Part model, mm, in its own coordinate system. A direction names the side the tool comes from. Give positions to 0.01 mm unless a question says otherwise; leave off trailing zeros. Write each loop counter-clockwise with the first axis right and the second up, starting at its lowest first coordinate (ties: lowest second). Pieces come first, ordered by that corner, then holes. Notation, with made-up numbers: (36, 73.25) - (51, 73.25) arc R23 ccw to (51, 84.25) - close; hole circle Ø3 at (72, -11.75). An arc over 180 degrees is marked (long way). Answer in a Markdown table with one row per item. Add a question column.
1. Which spindle directions (+Z, -Z, +X, -X, +Y, -Y) get a long thin tool onto all of the face, cutting with end or side? Do faces 1 (the cylindrical face through (41.727, 76.958, 23.918)), 2 (the cylindrical face through (57.14, 50.1, 19.34)), 3 (the flat face through (42, 47, 12)), 4 (the cylindrical face through (36.86, 50.1, 19.34)). Say none if no direction does.
2. Pull direction X, two halves, no side cores. Call faces 5 (the flat face through (41, 62, 18)), 6 (the cylindrical face through (43, 50, 26)), 7 (the cylindrical face through (36.86, 79.1, 18.18)): released by +X, released by -X, zero draft, split by the parting line, or undercut.
3. Drop flat-ended pins along their axis: pin 1 Ø4 at (y, z) = (55, 14) entering from -X; pin 2 Ø11 at (y, z) = (59, 15.5) entering from +X; pin 3 Ø8 at (x, y) = (48, 58.5) entering from +Z; pin 4 Ø1.8 at (x, y) = (41.5, 75.5) entering from -Z. Give the stop position or say it passes through.
4. Band-saw the part on A-A on z = 22. Write the cut outline in (x, y).
5. Band-saw the part on D-D on y = 56. Write the cut outline in (x, z).
6. Band-saw the part on B-B on x = 42. State how many separate pieces and enclosed holes the cut face has, plus the area to 3 significant figures.
7. Probe line 1 along Y through (x, z) = (54, 10.75); line 2 along X through (y, z) = (76, 10.25); line 3 along Y through (x, z) = (52, 28.5). List the from-to ranges inside material, lowest first.
```python
from build123d import *

# Parameters (mm, degrees)
CYLINDER027_R     = 0.8
CYLINDER027_DEPTH = 12
CYLINDER028_R     = 0.8
CYLINDER028_DEPTH = 12
CYLINDER029_R     = 0.8
CYLINDER029_DEPTH = 12
CYLINDER039_R     = 1
CYLINDER039_DEPTH = 45
CYLINDER040_R     = 2.1
CYLINDER040_DEPTH = 8
CYLINDER041_R     = 2.1
CYLINDER041_DEPTH = 8
CYLINDER026_R     = 0.8
CYLINDER026_DEPTH = 12
BOX043_W          = 2
BOX043_H          = 23
BOX043_DEPTH      = 13
BOX042_W          = 25
BOX042_H          = 21
BOX042_DEPTH      = 28
BOX030_W          = 22
BOX030_H          = 37
BOX030_DEPTH      = 26
FILLET002024_R    = 3
FILLET002034_R    = 3


with BuildPart() as obj1:
    # Cylinder027 → Cylinder027 (new body)
    with BuildSketch(Plane(origin=(54, 47, 0), x_dir=(1, 0, 0), z_dir=(0, 0, 1))):
        Circle(CYLINDER027_R)
    extrude(amount=CYLINDER027_DEPTH)


with BuildPart() as obj2:
    # Cylinder028 → Cylinder028 (new body)
    with BuildSketch(Plane(origin=(42, 76, 0), x_dir=(1, 0, 0), z_dir=(0, 0, 1))):
        Circle(CYLINDER028_R)
    extrude(amount=CYLINDER028_DEPTH)


with BuildPart() as obj3:
    # Cylinder029 → Cylinder029 (new body)
    with BuildSketch(Plane(origin=(54, 76, 0), x_dir=(1, 0, 0), z_dir=(0, 0, 1))):
        Circle(CYLINDER029_R)
    extrude(amount=CYLINDER029_DEPTH)


with BuildPart() as obj4:
    # Cylinder039 → Cylinder039 (new body)
    with BuildSketch(Plane(origin=(42, 40, 26), x_dir=(1, 0, 0), z_dir=(0, 1, 0))):
        Circle(CYLINDER039_R)
    extrude(amount=CYLINDER039_DEPTH)


with BuildPart() as obj5:
    # Cylinder040 → Cylinder040 (new body)
    with BuildSketch(Plane(origin=(42, 41, 26), x_dir=(1, 0, 0), z_dir=(0, 1, 0))):
        Circle(CYLINDER040_R)
    extrude(amount=CYLINDER040_DEPTH)


with BuildPart() as obj6:
    # Cylinder041 → Cylinder041 (new body)
    with BuildSketch(Plane(origin=(42, 74, 26), x_dir=(1, 0, 0), z_dir=(0, 1, 0))):
        Circle(CYLINDER041_R)
    extrude(amount=CYLINDER041_DEPTH)


with BuildPart() as fusion029:
    # Cylinder026 → Cylinder026 (new body)
    with BuildSketch(Plane(origin=(42, 47, 0), x_dir=(1, 0, 0), z_dir=(0, 0, 1))):
        Circle(CYLINDER026_R)
    extrude(amount=CYLINDER026_DEPTH)

    # Fusion029: union obj1, obj2, obj3, obj4, obj5, obj6
    add(obj1.part)
    add(obj2.part)
    add(obj3.part)
    add(obj4.part)
    add(obj5.part)
    add(obj6.part)


with BuildPart() as cube036:
    # Box043 → Box043 (new body)
    with BuildSketch(Plane(origin=(40.5, 50, 5), x_dir=(1, 0, 0), z_dir=(0, 0, 1))):
        with Locations((1, 11.5)):
            Rectangle(BOX043_W, BOX043_H)
    extrude(amount=BOX043_DEPTH)


with BuildPart() as cube035:
    # Box042 → Box042 (new body)
    with BuildSketch(Plane(origin=(35, 51, 8), x_dir=(1, 0, 0), z_dir=(0, 0, 1))):
        with Locations((12.5, 10.5)):
            Rectangle(BOX042_W, BOX042_H)
    extrude(amount=BOX042_DEPTH)


with BuildPart() as obj7:
    # Box030 → Box030 (new body)
    with BuildSketch(Plane(origin=(36, 43, 5), x_dir=(1, 0, 0), z_dir=(0, 0, 1))):
        with Locations((11, 18.5)):
            Rectangle(BOX030_W, BOX030_H)
    extrude(amount=BOX030_DEPTH)

    # Fillet002024
    fillet002024_edges = [obj7.edges().sort_by_distance(p)[0] for p in [
        (36, 43, 18),
        (36, 80, 18),
        (58, 43, 18),
        (58, 80, 18),
    ]]
    fillet(fillet002024_edges, radius=FILLET002024_R)

    # Cut007: cut Cube035
    add(cube035.part, mode=Mode.SUBTRACT)

    # Fusion028: union Cube036
    add(cube036.part)

    # Fillet002034
    fillet002034_edges = [obj7.edges().sort_by_distance(p)[0] for p in [
        (36, 51, 19.5),
        (36, 72, 19.5),
        (58, 51, 19.5),
        (58, 72, 19.5),
    ]]
    fillet(fillet002034_edges, radius=FILLET002034_R)

    # Cut008: cut Fusion029
    add(fusion029.part, mode=Mode.SUBTRACT)


solid = obj7.part
```
Values:
| question | item | result |
|---|---|---|
| 1 | face 1 | +Y |
| 1 | face 2 | +Z, +X |
| 1 | face 3 | -Z |
| 1 | face 4 | +Z, -X |
| 2 | face 5 | zero draft |
| 2 | face 6 | undercut |
| 2 | face 7 | released by -X |
| 3 | pin 1 | stops at x = 40.5 |
| 3 | pin 2 | stops at x = 42.5 |
| 3 | pin 3 | stops at z = 8 |
| 3 | pin 4 | stops at z = 5 |
| 4 | outline | (36, 46) arc R3 ccw to (39, 43) - (55, 43) arc R3 ccw to (58, 46) - (58, 48) arc R3 ccw to (55, 51) - (39, 51) arc R3 ccw to (36, 48) - close; (36, 75) arc R3 ccw to (39, 72) - (55, 72) arc R3 ccw to (58, 75) - (58, 77) arc R3 ccw to (55, 80) - (39, 80) arc R3 ccw to (36, 77) - close |
| 5 | outline | (36, 5) - (58, 5) - (58, 8) - (42.5, 8) - (42.5, 18) - (40.5, 18) - (40.5, 8) - (36, 8) - close |
| 6 | separate pieces | 3 |
| 6 | enclosed holes | 0 |
| 6 | area | 608 mm² |
| 7 | line 1 | y = 43 to 46.2, 47.8 to 51, 72 to 75.2, 76.8 to 80 |
| 7 | line 2 | x = 36 to 41.2, 42.8 to 53.2, 54.8 to 58 |
| 7 | line 3 | y = 43 to 51, 72 to 80 |
